Read the model definition and answer for the solid it produces. Units are mm, in the model's axes. A direction names the side the tool comes from. Round coordinates to 2 decimals unless told otherwise and drop trailing zeros. Order: outer loops, then holes, each group sorted by start corner. A loop starts at its lowest first (then second) coordinate and runs counter-clockwise, first axis right, second up. Notation, with made-up numbers: (-12, -11) - (1, -11) arc R27 ccw to (1, 28) - close; hole circle Ø6 at (-37.75, 32.25). An arc over 180 degrees is marked (long way). Answer as a JSON object with one key per item and string values. Group by question number.
Q1. A cutting plane is placed at A-A on y = 0. Determine the outline of the cut face in (x, z), and give its area (3 significant figures).
Q2. A cutting plane is placed at C-C on y = -1.75. Determine the outline of the cut face in (x, z).
Q3. A tool of negligible diameter and unlimited length cuts with its end or side. For faces 1 (the cylindrical face through (-3, 0, 10)), 2 (the flat face through (0, 0, 20)), from which of +Z, -Z, +X, -X, +Y, -Y can it reach the whole face along a straight path? Write none if from no direction.
Q4. A cutting plane is placed at B-B on z = 15. Determine the outline of the cut face in (x, y).
Q5. Consider line 1 (Y direction, x = 1.25, z = 13); line 2 (Y direction, x = 8.5, z = -11.5); line 3 (X direction, y = -1, z = 8). Determine where each line is inside the solid, lowest interval first.
Q6. Given pin 1 Ø4 at (x, z) = (1.5, 13.5) entering from +Y; pin 2 Ø6 at (x, z) = (13.5, -1) entering from -Y; pin 3 Ø1.5 at (y, z) = (1.5, -8.5) entering from +X; pin 4 Ø2 at (x, y) = (9.5, 1.5) entering from +Z, each flat-ended and moving along its own axis, determine where each tip first touches the part or whether it passes through.
```python
from build123d import *

# Parameters (mm, degrees)
TORUS_R               = 3
TORUS_ANGLE           = 125
TORUS_ROLL_ANGLE      = -90
TORUS_PLACEMENT_ANGLE = 180
CYLINDER_R            = 3
CYLINDER_DEPTH        = 20


with BuildPart() as torus:
    # Torus → Torus (revolve)
    with BuildSketch(Plane.XZ):
        with Locations((10, 0)):
            Circle(TORUS_R)
    revolve(axis=Axis((0, 0, 0), (0, 0, 1)), revolution_arc=TORUS_ANGLE)


with BuildPart() as torus_1:
    # Torus roll: moved
    add(torus.part.rotate(Axis((0, 0, 0), (1, 0, 0)), TORUS_ROLL_ANGLE))


with BuildPart() as torus_2:
    # Torus placement: moved
    add(torus_1.part.moved(Location((10, 0, 0))).rotate(Axis((10, 0, 0), (0, 0, 1)), TORUS_PLACEMENT_ANGLE))


with BuildPart() as fusion:
    # Cylinder → Cylinder (new body)
    with BuildSketch(Plane.XY):
        Circle(CYLINDER_R)
    extrude(amount=CYLINDER_DEPTH)

    # Fusion: union Torus
    add(torus_2.part)


solid = fusion.part
```
Result set:
{
 "1": {"outline": "(-3, 0) arc R13 ccw to (17.46, -10.65) - (14.02, -5.73) arc R7 cw to (3, 0) - (3, 20) - (-3, 20) - close", "area": "251 mm²"},
 "2": {"outline": "(-2.44, 0) arc R12.44 ccw to (17.13, -10.19) - (14.34, -6.2) arc R7.56 cw to (2.44, 0) - (2.44, 20) - (-2.44, 20) - close"},
 "3": {"face 1": "+Z", "face 2": "+Z, +X, -X, +Y, -Y"},
 "4": {"outline": "circle Ø6 at (0, 0)"},
 "5": {"line 1": "y = -2.73 to 2.73", "line 2": "y = -2.54 to 2.54", "line 3": "x = -2.83 to 2.83"},
 "6": {"pin 1": "stops at y = 3", "pin 2": "passes through", "pin 3": "stops at x = 16.48", "pin 4": "stops at z = -7"}
}
